Model file for the job. Use its own axes, mm. Face numbers are marked on the shaded views. A direction names the side the tool comes from. Coordinates: 2 decimals unless noted, no trailing zeros. Write each loop counter-clockwise with the first axis right and the second up, starting at its lowest first coordinate (ties: lowest second). Pieces come first, ordered by that corner, then holes. Notation, with made-up numbers: M -18,86.5 L 11,86.5 A21 ccw 11,111.5 Z; hole C 52.5,21.25 d9. An arc over 180 degrees is marked long. Put each result on its own line as item: value. Start each with the question number.
Q1. Which spindle directions (+Z, -Z, +X, -X, +Y, -Y) get a long thin tool onto all of the face, cutting with end or side? Do the marked faces 5, 6, 7 and 8. Say none if no direction does.
Q2. Drop flat-ended pins along their axis: pin 1 (6 mm diameter, centred on x = 5, y = 6.5, fed in from -Z); pin 2 (4 mm diameter, centred on x = 23, z = 6, fed in from -Y); pin 3 (4 mm diameter, centred on x = 13.5, z = 5.5, fed in from -Y); pin 4 (4 mm diameter, centred on x = 8, y = 6.5, fed in from -Z). Give the stop position or say it passes through.
Q3. Pull direction Y, two halves, no side cores. Call the marked faces 1, 2, 3 and 4: pulls with the +Y half, pulls with the -Y half, needs draft (parallel to the pull), parting line crosses it, or undercut.
Q4. Cut at D-D (y = -10.5). Write the cut outline in (x, z), then the cut area to 3 significant figures.
Q5. Cut at A-A (x = 0). Write the cut outline in (y, z).
Q6. Cut at C-C (z = 6.25). Write the cut outline in (x, y), then the cut area to 3 significant figures.
Q7. Cut at B-B (y = 0). Write the cut outline in (x, z).
Q8. Drill centre lines: line 1 along Z through (x, y) = (3, 5); line 2 along X through (y, z) = (6, 7.25); line 3 along Y through (x, z) = (-9, 10.75). Where is each one in solid material? Low to high.
Autodesk Inventor part; units mm, degrees
ref_plane "РабПлоскость1" through (-24.7024, -23.7395, 10.5) normal (0, 0, 1) x (1, 0, 0)
ref_plane "РабПлоскость2" through (-24.7024, -23.7395, 9) normal (0, 0, -1) x (0, 1, 0)
ref_plane "YZ Plane" through (0, 0, 0) normal (1, 0, 0) x (0, 1, 0)
sketch "Эскиз1" plane through (0, 0, 0) normal (0, 0, 1) x (1, 0, 0)
  line L0 (0, 0) -> (34.5691, 5.4752) construction
  line L1 (0, 0) -> (35, 0) construction
  line L2 (0, 0) -> (34.5691, -5.4752) construction
  circle A0 centre (0, 0) radius 11.25
  circle A1 centre (0, 0) radius 15
  circle A2 centre (0, 0) radius 20
  circle A3 centre (0, 0) radius 30.0525
  circle A4 centre (0, 0) radius 32.0038
  circle A5 centre (0, 0) radius 35
  line L3 (0, 0) -> (17.5, -30.3109) construction
  circle A6 centre (0, -8) radius 1.5
  circle A7 centre (-8, 0) radius 1.5
  line L4 (0, 0) -> (-35, 0) construction
  line L5 (-29.6307, -4.693) -> (-19.4416, -4.693) construction
  line L6 (-29.6307, -4.693) -> (-19.4416, -4.693)
  line L7 (-29.6839, -4.693) -> (-29.6839, 4.693)
  line L8 (-19.4416, 4.693) -> (-34.6839, 4.693) construction
  line L9 (-19.4416, -4.693) -> (-34.6839, -4.693) construction
  line L10 (10.751, 28.0074) -> (5.6565, 19.1834) construction
  line L11 (5.6565, 19.1834) -> (13.2777, 32.3837) construction
  line L12 (-5.6565, 19.1834) -> (-13.2777, 32.3837) construction
  circle A8 centre (0, 8) radius 1.5
  line L13 (0, 0) -> (-17.5, 30.3109) construction
  line L14 (-5.6565, 19.1834) -> (-13.2777, 32.3837)
  line L15 (0, 0) -> (17.5, 30.3109) construction
  line L16 (0, 0) -> (-17.5, -30.3109) construction
  line L17 (5.6565, 19.1834) -> (13.2777, 32.3837)
  line L18 (13.3758, 26.5536) -> (16.0133, 31.1219)
  line L19 (16.3082, 24.8605) -> (18.9457, 29.4289)
  line L20 (18.9457, 29.4289) -> (17.4457, 26.8308) construction
  line L21 (29.6307, 4.693) -> (19.4416, 4.693)
  line L22 (18.8796, -23.3144) -> (13.7851, -14.4904) construction
  line L23 (13.7851, -14.4904) -> (21.4063, -27.6907) construction
  line L24 (29.6839, 4.693) -> (29.6839, 1.693)
  line L25 (29.6839, 4.693) -> (29.6839, -4.693)
  line L26 (29.6839, -4.693) -> (29.6839, -1.693) construction
  circle A9 centre (8, 0) radius 1.5
  line L27 (-18.8796, 23.3144) -> (-13.7851, 14.4904) construction
  line L28 (-13.7851, 14.4904) -> (-21.4063, 27.6907) construction
  line L29 (-18.8796, 23.3144) -> (-13.7851, 14.4904)
  line L30 (-13.7851, 14.4904) -> (-21.4063, 27.6907)
  line L31 (-18.9063, 23.3605) -> (-10.7777, 28.0536)
  line L32 (-16.3082, 24.8605) -> (-18.9457, 29.4289)
  line L33 (-13.3758, 26.5536) -> (-16.0133, 31.1219)
  line L34 (-13.7851, -14.4904) -> (-21.4063, -27.6907) construction
  line L35 (-10.751, -28.0074) -> (-5.6565, -19.1834) construction
  line L36 (-13.7851, -14.4904) -> (-21.4063, -27.6907)
  line L37 (-10.751, -28.0074) -> (-5.6565, -19.1834)
  line L38 (13.7851, 14.4904) -> (21.4063, 27.6907) construction
  line L39 (21.4063, 27.6907) -> (20.1674, 25.5449) construction
  line L40 (10.7777, 28.0536) -> (18.9063, 23.3605)
  line L41 (13.7851, 14.4904) -> (21.4063, 27.6907)
  line L42 (10.751, 28.0074) -> (5.6565, 19.1834)
  line L43 (0, 0) -> (21.2118, 27.8399) construction
  line L44 (0, 0) -> (8, 0) construction
  line L45 (0, 0) -> (0, 8) construction
  line L46 (-10.7777, -28.0536) -> (-18.9063, -23.3605)
  line L47 (-13.3758, -26.5536) -> (-16.0133, -31.1219)
  line L48 (-16.3082, -24.8605) -> (-18.9457, -29.4289)
  line L49 (-5.6565, -19.1834) -> (-13.2777, -32.3837) construction
  line L50 (5.6565, -19.1834) -> (13.2777, -32.3837) construction
  line L51 (-5.6565, -19.1834) -> (-13.2777, -32.3837)
  line L52 (18.8796, -23.3144) -> (13.7851, -14.4904)
  line L53 (5.6565, -19.1834) -> (13.2777, -32.3837)
  line L54 (16.3082, -24.8605) -> (18.9457, -29.4289)
  line L55 (13.7851, -14.4904) -> (21.4063, -27.6907)
  line L56 (13.3758, -26.5536) -> (16.0133, -31.1219)
  line L57 (18.9063, -23.3605) -> (10.7777, -28.0536)
  line L58 (27.6414, 16.1308) -> (28.831, 19.8437)
  line L59 (24.938, 20.0584) -> (28.831, 19.8437)
  line L60 (24.7499, 20.2901) -> (25.3388, 24.1443)
  line L61 (21.4607, 23.742) -> (25.3388, 24.1443)
  line L62 (17.4457, 26.8308) -> (21.2118, 27.8399)
  line L63 (21.2384, 23.9411) -> (21.2118, 27.8399)
  line L64 (-19.4416, 4.693) -> (-34.6839, 4.693)
  line L65 (-17.4453, 26.8311) -> (-21.2113, 27.8403)
  line L66 (-21.238, 23.9415) -> (-21.2113, 27.8403)
  line L67 (-21.4603, 23.7424) -> (-25.3384, 24.1447)
  line L68 (-24.7496, 20.2905) -> (-25.3384, 24.1447)
  line L69 (-24.9377, 20.0588) -> (-28.8307, 19.8442)
  line L70 (-27.6411, 16.1312) -> (-28.8307, 19.8442)
  line L71 (-27.7903, 15.8727) -> (-31.6007, 15.0465)
  line L72 (-29.8401, 11.5678) -> (-31.6007, 15.0465)
  line L73 (-29.9467, 11.289) -> (-33.5789, 9.8719)
  line L74 (-31.2916, 6.7145) -> (-33.5789, 9.8719)
  line L75 (-31.3528, 6.4224) -> (-34.716, 4.45)
  line L76 (-29.6839, -1.693) -> (-34.959, -1.693)
  line L77 (-19.4416, -4.693) -> (-34.6839, -4.693)
  line L78 (-29.6839, 1.693) -> (-34.959, 1.693)
  line L79 (-31.959, 1.693) -> (-34.716, 4.45)
  line L80 (-31.9591, -1.6925) -> (-34.716, -4.4494)
  line L81 (-31.3529, -6.4219) -> (-34.716, -4.4494)
  line L82 (-31.2917, -6.714) -> (-33.5791, -9.8714)
  line L83 (-29.9469, -11.2885) -> (-33.5791, -9.8714)
  line L84 (-29.8403, -11.5673) -> (-31.6009, -15.046)
  line L85 (-27.7906, -15.8723) -> (-31.6009, -15.046)
  line L86 (-24.938, -20.0584) -> (-28.831, -19.8437)
  line L87 (-27.6414, -16.1308) -> (-28.831, -19.8437)
  line L88 (-17.4457, -26.8308) -> (-21.2118, -27.8399)
  line L89 (-21.2384, -23.9411) -> (-21.2118, -27.8399)
  line L90 (-21.4607, -23.742) -> (-25.3388, -24.1443)
  line L91 (-24.7499, -20.2901) -> (-25.3388, -24.1443)
  line L92 (-14.5138, -28.5236) -> (-13.5047, -32.2897)
  line L93 (-10.1149, -30.3634) -> (-13.5047, -32.2897)
  line L94 (-9.8313, -30.4564) -> (-8.2407, -34.016)
  line L95 (-5.1973, -31.579) -> (-8.2407, -34.016)
  line L96 (-4.9026, -31.6261) -> (-2.7702, -34.8902)
  line L97 (-0.1495, -32.0035) -> (-2.7702, -34.8902)
  line L98 (0.149, -32.0035) -> (2.7697, -34.8902)
  line L99 (-14.5133, 28.5238) -> (-13.5042, 32.2899)
  line L100 (-10.1144, 30.3635) -> (-13.5042, 32.2899)
  line L101 (-9.8308, 30.4565) -> (-8.2401, 34.0162)
  line L102 (-5.1968, 31.5791) -> (-8.2401, 34.0162)
  line L103 (14.5138, 28.5236) -> (13.5047, 32.2897)
  line L104 (10.1149, 30.3634) -> (13.5047, 32.2897)
  line L105 (9.8313, 30.4564) -> (8.2407, 34.016)
  line L106 (5.1973, 31.579) -> (8.2407, 34.016)
  line L107 (4.9026, 31.6261) -> (2.7702, 34.8902)
  line L108 (0.1495, 32.0035) -> (2.7702, 34.8902)
  line L109 (-4.9021, 31.6262) -> (-2.7697, 34.8902)
  line L110 (-0.149, 32.0035) -> (-2.7697, 34.8902)
  line L111 (14.5133, -28.5238) -> (13.5042, -32.2899)
  line L112 (5.1968, -31.5791) -> (8.2401, -34.0162)
  line L113 (9.8308, -30.4565) -> (8.2401, -34.0162)
  line L114 (10.1144, -30.3635) -> (13.5042, -32.2899)
  line L115 (17.4453, -26.8311) -> (21.2113, -27.8403)
  line L116 (21.238, -23.9415) -> (21.2113, -27.8403)
  line L117 (4.9021, -31.6262) -> (2.7697, -34.8902)
  line L118 (19.4416, -4.693) -> (34.6839, -4.693)
  line L119 (29.6839, -1.693) -> (34.959, -1.693)
  line L120 (21.4603, -23.7424) -> (25.3384, -24.1447)
  line L121 (24.7496, -20.2905) -> (25.3384, -24.1447)
  line L122 (24.9377, -20.0588) -> (28.8307, -19.8442)
  line L123 (27.6411, -16.1312) -> (28.8307, -19.8442)
  line L124 (27.7903, -15.8727) -> (31.6007, -15.0465)
  line L125 (29.9467, -11.289) -> (33.5789, -9.8719)
  line L126 (31.2916, -6.7145) -> (33.5789, -9.8719)
  line L127 (31.3528, -6.4224) -> (34.716, -4.45)
  line L128 (31.959, -1.693) -> (34.716, -4.45)
  line L129 (29.8401, -11.5678) -> (31.6007, -15.0465)
  line L130 (34.5691, 5.4752) -> (29.6307, 4.693) construction
  line L131 (19.4416, 4.693) -> (34.6839, 4.693)
  line L132 (34.6839, 4.693) -> (29.6839, 4.693) construction
  line L133 (29.6839, 1.693) -> (34.959, 1.693)
  line L134 (29.8403, 11.5673) -> (31.6009, 15.046)
  line L135 (31.2917, 6.714) -> (33.5791, 9.8714)
  line L136 (31.9591, 1.6925) -> (34.716, 4.4494)
  line L137 (31.3529, 6.4219) -> (34.716, 4.4494)
  line L138 (29.9469, 11.2885) -> (33.5791, 9.8714)
  line L139 (27.7906, 15.8723) -> (31.6009, 15.046)
  circle A10 centre (0, 0) radius 36.5
  line L140 (0, 0) -> (-24.7487, 24.7487) construction
  line L141 (0, 0) -> (35, 0) construction
  line L142 (0, 0) -> (-24.6962, 0) construction
  line L143 (-24.6962, -4.693) -> (-24.6962, 4.693)
  line L144 (-8.2838, -23.734) -> (-16.4124, -19.041)
  line L145 (16.4124, -19.041) -> (8.2838, -23.734)
  line L146 (24.6962, 4.693) -> (24.6962, -4.693)
  line L147 (8.2838, 23.734) -> (16.4124, 19.041)
  line L148 (-16.4124, 19.041) -> (-8.2838, 23.734)
  line L149 (0, 0) -> (21.2503, 21.2503) construction
  line L150 (0, 0) -> (30.0525, 0) construction
  line L151 (14.1421, 14.1421) -> (23.5912, 4.693)
  line L152 (23.5912, 4.693) -> (-6.168, 34.4522)
  point P0 (0, 0)
  point P1 (18.9062, 23.3604)
  point P2 (18.9055, 23.3609)
  point P3 (10.7784, 28.0531)
  point P4 (-10.7784, 28.0531)
  point P5 (-18.9055, 23.3609)
  point P6 (-18.9062, 23.3604)
  point P7 (-29.6838, 4.693)
  point P8 (-29.6839, 4.6922)
  point P9 (-29.6839, -4.6922)
  point P10 (-18.9055, -23.3609)
  point P11 (-10.7784, -28.0531)
  point P12 (-10.7776, -28.0534)
  point P13 (10.7776, -28.0534)
  point P14 (10.7784, -28.0531)
  point P15 (18.9055, -23.3609)
  point P16 (29.6839, -4.6922)
  point P17 (29.6839, 4.6922)
  point P18 (29.6838, 4.693)
  point P19 (-29.6838, -4.693)
  point P20 (-18.9062, -23.3604)
  point P21 (18.9062, -23.3604)
  point P22 (29.6838, -4.693)
  point P23 (10.7776, 28.0534)
  point P24 (-10.7776, 28.0534)
  point P25 (-24.6962, 4.693)
  point P26 (24.6962, -4.693)
  dimension "d10" = 70
  dimension "d21" = 60.105
  dimension "d11" = 40
  dimension "d12" = 9
  dimension "d13" = 5
  dimension "d14" = 360
  dimension "d15" = 360
  dimension "d16" = 5
  dimension "d17" = 90
  dimension "d18" = 3
  dimension "d19" = 3
  dimension "d20" = 360
  dimension "d22" = 3
  dimension "d23" = 45
  dimension "d24" = 45.392
  dimension "d25" = 360
  dimension "d26" = 22.5
  dimension "d27" = 8
  dimension "d28" = 3
  dimension "d29" = 8
  dimension "d30" = 3
  dimension "d31" = 30
  dimension "d32" = 73
  dimension "d45" = 135
  dimension "d48" = 360
  dimension "d54" = 45
extrude "Выдавливание1" add sketch "Эскиз1" along normal blind 10.5 contours A1 | A2
extrude "Выдавливание4" add sketch "Эскиз1" along normal blind 1 from surface at 10.5 contours A0 | A1 | A2
ref_plane "РабПлоскость1" through (-24.7024, -23.7395, 10.5) normal (0, 0, 1) x (1, 0, 0)
ref_plane "РабПлоскость2" through (-24.7024, -23.7395, 9) normal (0, 0, -1) x (0, 1, 0)
extrude "Выдавливание7" add sketch "Эскиз1" along normal blind 11.5 contours A2 L21 L146 L118 | L52 L145 L53 A2 | A2 L17 L152 L41 | L152 L17 L147 L41 | L37 L144 L36 A2 | A2 L29 L148 L14 | L6 L143 L64 A2
ref_plane "РабПлоскость3" through (23.5912, 4.693, 0) normal (0.7071068, 0.7071068, 0) x (-0.7071068, 0.7071068, 0)
sketch "Эскиз2" plane through (23.5912, 4.693, 0) normal (0.7071068, 0.7071068, 0) x (-0.7071068, 0.7071068, 0)
  line L0 (13.363, 0) -> (13.363, 3.5)
  line L1 (13.8618, 0) -> (13.8618, 11.5)
  line L2 (13.363, 0) -> (16.863, 0) construction
  circle A0 centre (13.363, 3.5) radius 2
  dimension "d56" = 3.5
  dimension "d57" = 90
  dimension "d58" = 4
extrude "Выдавливание8" cut sketch "Эскиз2" along normal blind 5.1 and the other way blind 9
properties part number "inside_part_wheel"
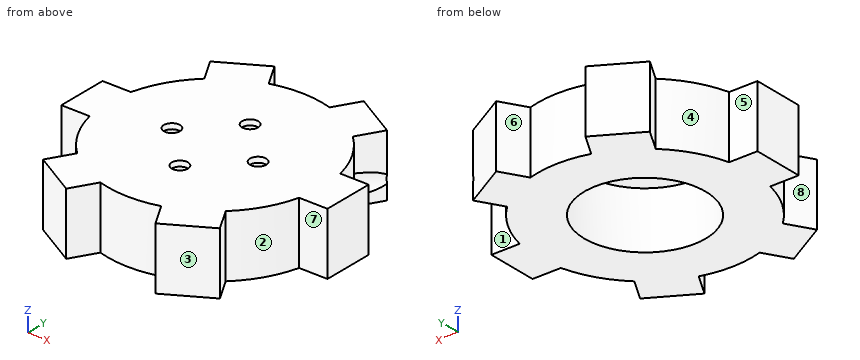
Computed values:
1. face 5: +Z, -Z, -X, +Y
1. face 6: +Z, -Z, +Y
1. face 7: +Z, -Z, +X, -Y
1. face 8: +Z, -Z, -X
2. pin 1: z = 10.5
2. pin 2: y = -4.69
2. pin 3: y = -21.88
2. pin 4: z = 0
3. face 1: pulls with the +Y half
3. face 2: undercut
3. face 3: pulls with the -Y half
3. face 4: undercut
4. outline: M -17.02,0 L -4.04,0 L -4.04,10.5 L 4.04,10.5 L 4.04,0 L 17.02,0 L 17.02,11.5 L -17.02,11.5 Z
4. area: 307 mm2
5. outline: M -20,0 L -11.25,0 L -11.25,10.5 L -9.5,10.5 L -9.5,11.5 L -20,11.5 Z; M -6.5,10.5 L 6.5,10.5 L 6.5,11.5 L -6.5,11.5 Z; M 9.5,10.5 L 11.25,10.5 L 11.25,0 L 20,0 L 20,11.5 L 9.5,11.5 Z
6. outline: M -24.7,-4.69 L -19.44,-4.69 A20 ccw -13.79,-14.49 L -16.41,-19.04 L -8.28,-23.73 L -5.66,-19.18 A20 ccw 5.66,-19.18 L 8.28,-23.73 L 16.41,-19.04 L 13.79,-14.49 A20 ccw 19.44,-4.69 L 24.7,-4.69 L 24.7,4.69 L 19.44,4.69 A20 ccw 13.79,14.49 L 16.41,19.04 L 8.28,23.73 L 5.66,19.18 A20 ccw -5.66,19.18 L -8.28,23.73 L -16.41,19.04 L -13.79,14.49 A20 ccw -19.44,4.69 L -24.7,4.69 Z; hole C 0,0 d22.5
6. area: 1,130 mm2
7. outline: M -24.7,0 L -11.25,0 L -11.25,10.5 L -9.5,10.5 L -9.5,11.5 L -24.7,11.5 Z; M -6.5,10.5 L 6.5,10.5 L 6.5,11.5 L -6.5,11.5 Z; M 9.5,10.5 L 11.25,10.5 L 11.25,0 L 24.7,0 L 24.7,11.5 L 9.5,11.5 Z
8. line 1: 10.5 to 11.5
8. line 2: -19.08 to -9.52, 9.52 to 19.08
8. line 3: -23.32 to -1.12, 1.12 to 23.32
